Autodesk Inventor part; units mm, degrees
ref_plane "YZ Plane" through (0, 0, 0) normal (1, 0, 0) x (0, 1, 0)
ref_plane "XZ Plane" through (0, 0, 0) normal (0, 1, 0) x (-1, 0, 0)
ref_plane "XY Plane" through (0, 0, 0) normal (0, 0, 1) x (1, 0, 0)
sketch "Sketch1" plane through (0, 0, 0) normal (0, 0, 1) x (1, 0, 0)
  circle A0 centre (0, 0) radius 14.2875
  circle A1 centre (0, 0) radius 20.6375
  circle A2 centre (0, -31.75) radius 4.7625
  circle A3 centre (-19.05, 29.2721) radius 4.7625
  circle A4 centre (19.05, 29.2721) radius 4.7625
  arc A5 (-23.7912, 29.7223) -> (-3.6429, -34.8176) centre (63.1904, 21.4615) ccw
  arc A6 (3.6429, -34.8176) -> (23.7912, 29.7223) centre (-63.1904, 21.4615) ccw
  arc A7 (-14.5681, 30.8826) -> (14.5681, 30.8826) centre (0, 36.1176) ccw
  dimension "d0" = 28.575
  dimension "d1" = 6.35
  dimension "d2" = 9.525
  dimension "d3" = 9.525
  dimension "d4" = 9.525
  dimension "d7" = 6.35
  dimension "d8" = 9.525
  dimension "d9" = 9.525
  dimension "d13" = 19.05
extrude "Extrusion1" add sketch "Sketch1" against normal blind 6.35
hole "Hole1" at (0, 0, 0) at (-19.05, 29.2721, 0) at (19.05, 29.2721, 0) at (0, -31.75, 0) direction (0, 0, -1) diameter 5.1054 end through all
properties part number "GP5-027" material "Aluminum 6061"
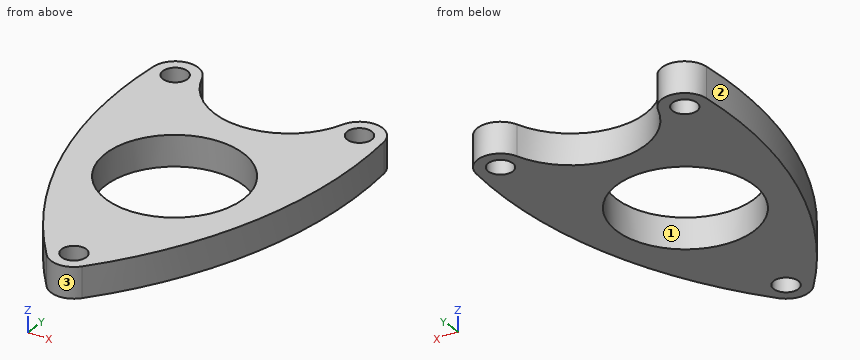
Input: part model. Units: mm. Frame: model coordinates. Face numbers are marked on the shaded views. Round coordinates to 2 decimals unless told otherwise and drop trailing zeros. Write each loop counter-clockwise with the first axis right and the second up, starting at its lowest first coordinate (ties: lowest second). Pieces come first, ordered by that corner, then holes. Notation, with made-up numbers: M 83,89 L 131,89 A25 cw 131,127 Z; hole C 7,12.5 d8. An arc over 180 degrees is marked long. Write each question's results on one line, items separated by ' | '.
Q1. Section query D-D (x = -5.5). Return loops of the section in (y, z).
Results:
outline: M -32.54,-6.35 L -13.19,-6.35 L -13.19,0 L -32.54,0 Z; M 13.19,-6.35 L 21.65,-6.35 L 21.65,0 L 13.19,0 Z
Q2. Section query B-B (y = 29). Return loops of the section in (x, z).
Results:
outline: M -23.86,-6.35 L -21.59,-6.35 L -21.59,0 L -23.86,0 Z; M -16.51,-6.35 L -13.75,-6.35 L -13.75,0 L -16.51,0 Z; M 13.75,-6.35 L 16.51,-6.35 L 16.51,0 L 13.75,0 Z; M 21.59,-6.35 L 23.86,-6.35 L 23.86,0 L 21.59,0 Z
Q3. Draft query along X for the marked faces 1, 2 and 3. Return one class per face: released by +X, released by -X, zero draft, split by the parting line, or undercut.
Results:
face 1: undercut | face 2: released by -X | face 3: split by the parting line
Q4. Line query: line 1 along Y through (x, z) = (0, -1.25); line 2 along X through (y, z) = (28.5, -4.5); line 3 along X through (y, z) = (-7.5, -5.25). Output: solid intervals per line, ascending.
Results:
line 1: y = -36.51 to -34.3, -29.2 to -14.29, 14.29 to 20.64 | line 2: x = -23.9 to -21.48, -16.62 to -13.48, 13.48 to 16.62, 21.48 to 23.9 | line 3: x = -19.24 to -12.16, 12.16 to 19.24
Q5. Section query C-C (z = -2). State how many separate pieces and enclosed holes the cut face has, and give its area (3 significant figures).
Results:
separate pieces: 1 | enclosed holes: 4 | area: 1,570 mm^2
Q6. Section query A-A (x = 0). Return loops of the section in (y, z).
Results:
outline: M -36.51,-6.35 L -34.3,-6.35 L -34.3,0 L -36.51,0 Z; M -29.2,-6.35 L -14.29,-6.35 L -14.29,0 L -29.2,0 Z; M 14.29,-6.35 L 20.64,-6.35 L 20.64,0 L 14.29,0 Z
Q7. Pin query (flat end, axial travel): P1, Ø3, axis at x = 0, y = -31.75, coming from the +Z side. Return the tip coordinate at first contact, or that it passes through.
Results:
P1: passes through
